For this review, take the finished solid that the model builds, in its own axes (mm). Face numbers are marked on the shaded views. A direction names the side the tool comes from. Coordinates: 2 decimals unless noted, no trailing zeros. Loops run counter-clockwise (first coordinate to the right, second up) from the corner with the lowest first, then second, coordinate; pieces in that order, holes last.
1. Take a section at A-A, the plane x = 65. Count the separate pieces of the cut face and the enclosed holes in it, then the cut area to 3 significant figures.
2. Clearance check with flat-ended pins moving along their axes: P1, Ø14.5, axis at y = 9.5, z = -78, coming from the -X side; P2, Ø1, axis at x = 55.5, y = 88, coming from the +Z side; P3, Ø4.5, axis at x = 42, y = 48, coming from the -Z side. State where each tip first meets the part, or that it passes through.
3. Take a section at B-B, the plane z = 59.5. State the section outline as (x, y) points, then the cut area to 3 significant figures.
4. Take a section at D-D, the plane z = -88. State the section outline as (x, y) points.
5. To check wall thickness, follow probe 1 along X at (y, z) = (13, 30); probe 2 along X at (y, z) = (11, -58); probe 3 along X at (y, z) = (12, -79). State the ranges of each line that lie inside material, in increasing order.
6. Machinability: for the marked faces 1, 2, 3 and 4, which of the approach directions +Z, -Z, +X, -X, +Y, -Y give a long, thin tool a straight path to every point of the face, cutting with its end or side? Answer none if there is none.
7. Take a section at C-C, the plane y = 47. State the section outline as (x, z) points, then the cut area to 3 significant figures.
8. Mouldability with a two-part tool opening along X and no side actions: class the marked faces 5, 6 and 7 as pulls with the +X half, pulls with the -X half, needs draft (parallel to the pull), parting line crosses it, or undercut.
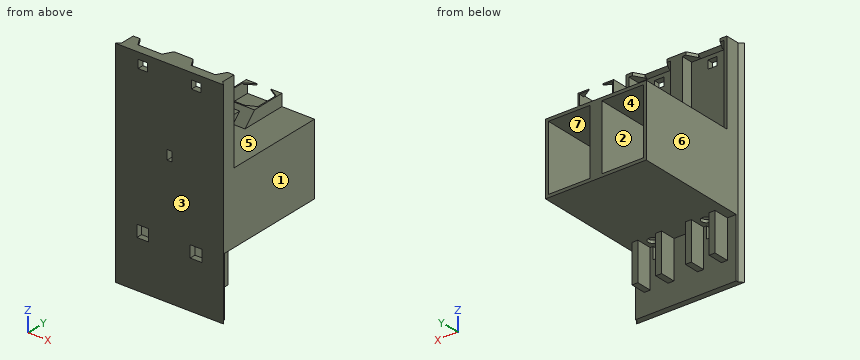
```python
from build123d import *

# Parameters (mm, degrees)
SKETCH1_W                                 = 85
SKETCH1_H                                 = 60
BOSS_EXTRUDE1_DEPTH                       = 100
CUT_EXTRUDE1_START                        = 5
SKETCH2_W                                 = 35
SKETCH2_H                                 = 55
CUT_EXTRUDE1_DEPTH                        = 95
SKETCH3_W                                 = 85
SKETCH3_H                                 = 5
BOSS_EXTRUDE2_DEPTH                       = 70
BOSS_EXTRUDE3_DEPTH                       = 10
SKETCH5_W                                 = 20
SKETCH5_H                                 = 2.5
CUT_EXTRUDE2_DEPTH                        = 7.5
SKETCH6_W                                 = 35
SKETCH6_H                                 = 12
CUT_EXTRUDE4_DEPTH                        = 57.5
CUT_EXTRUDE6_REACH                        = 186.73
SKETCH7_R                                 = 4
SKETCH9_W                                 = 85
SKETCH9_H                                 = 50
BOSS_EXTRUDE4_DEPTH                       = 5
SKETCH13_W                                = 8
SKETCH13_H                                = 7
CUT_EXTRUDE8_BUTTON_HOLES_DEPTH           = 169.374582405
BOSS_EXTRUDE5_OLED_MOUNT_DEPTH            = 10
BOSS_EXTRUDE6_OLED_MOUNT_DEPTH            = 1
BOSS_EXTRUDE7_START                       = -2.5
BOSS_EXTRUDE7_OLED_MOUNT_DEPTH            = 1
BOSS_EXTRUDE8_OLED_MOUNT_DEPTH            = 1
BOSS_EXTRUDE13_OLED_MOUNT_SUPPORT_DEPTH   = 30
CUT_EXTRUDE9_OLED_CABLE_DEPTH             = 10
CUT_EXTRUDE9_OLED_CABLE_DEPTH_BACK        = 157.553505231
SKETCH18_W                                = 4
SKETCH18_H                                = 8
BOSS_EXTRUDE12_OLED_CABLE_GUIDE_REACH     = 164.942
SKETCH20_W                                = 10
SKETCH20_H                                = 10
CUT_EXTRUDE10_SOLENOID_WIRE_HOLE_DEPTH    = 169.374582405
SKETCH21_W                                = 5
SKETCH21_H                                = 32
BOSS_EXTRUDE9_SOLENOID_SIDE_SUPPORT_DEPTH = 13
CHAMFER3_THUMB_SIZE                       = 2.5
CHAMFER5_THUMB_SIZE                       = 4.5
CHAMFER5_THUMB_SIZE2                      = 7.794228634
CHAMFER5_THUMB_PART_2_SIZE                = 4.5
CHAMFER5_THUMB_PART_2_SIZE2               = 7.794228634
CHAMFER5_THUMB_PART_3_SIZE                = 4.5
CHAMFER5_THUMB_PART_3_SIZE2               = 7.794228634
BOSS_EXTRUDE5_GUIDE_DEPTH                 = 180
SKETCH49_W                                = 10
SKETCH49_H                                = 10
BOSS_EXTRUDE14_DEPTH                      = 10
CHAMFER8_SIZE                             = 10


with BuildPart() as part:
    # Sketch1 → Boss-Extrude1 (new body)
    with BuildSketch(Plane(origin=(0, 0, 0), x_dir=(1, 0, 0), z_dir=(0, 1, 0))):
        with Locations((42.5, 30)):
            Rectangle(SKETCH1_W, SKETCH1_H)
    extrude(amount=BOSS_EXTRUDE1_DEPTH)

    # Sketch2 → Cut-Extrude1 (cut)
    with BuildSketch(Plane(origin=(0, 0, 0), x_dir=(1, 0, 0), z_dir=(0, 1, 0)).offset(CUT_EXTRUDE1_START)):
        with Locations((20, 30)):
            Rectangle(SKETCH2_W, SKETCH2_H)
        with Locations((65, 30)):
            Rectangle(SKETCH2_W, SKETCH2_H)
    extrude(amount=CUT_EXTRUDE1_DEPTH, mode=Mode.SUBTRACT)

    # Sketch3 → Boss-Extrude2 (add)
    with BuildSketch(Plane.XY):
        with Locations((42.5, 2.5)):
            Rectangle(SKETCH3_W, SKETCH3_H)
    extrude(amount=BOSS_EXTRUDE2_DEPTH)

    # Sketch4 → Boss-Extrude3 (add)
    with BuildSketch(Plane(origin=(0, 5, 0), x_dir=(1, 0, 0), z_dir=(0, 1, 0))):
        Polygon((85, 0), (82.5, 0), (82.5, -67.5), (47.5, -67.5), (47.5, 0), (37.5, 0), (37.5, -67.5), (2.5, -67.5), (2.5, 0), (0, 0), (0, -70), (85, -70), align=None)
    extrude(amount=BOSS_EXTRUDE3_DEPTH)

    # Sketch5 → Cut-Extrude2 (cut)
    with BuildSketch(Plane(origin=(0, 15, 0), x_dir=(1, 0, 0), z_dir=(0, 1, 0))):
        with Locations((20, -68.75)):
            Rectangle(SKETCH5_W, SKETCH5_H)
        with Locations((65, -68.75)):
            Rectangle(SKETCH5_W, SKETCH5_H)
    extrude(amount=-CUT_EXTRUDE2_DEPTH, mode=Mode.SUBTRACT)

    # Sketch6 → Cut-Extrude4 (cut)
    with BuildSketch(Plane.XY):
        with Locations((20, 11)):
            Rectangle(SKETCH6_W, SKETCH6_H)
        with Locations((65, 11)):
            Rectangle(SKETCH6_W, SKETCH6_H)
    extrude(amount=-CUT_EXTRUDE4_DEPTH, mode=Mode.SUBTRACT)

    # Sketch7 → Cut-Extrude6 (cut, up to next)
    with BuildSketch(Plane(origin=(0, 0, -60), x_dir=(-1, 0, 0), z_dir=(0, 0, -1)), mode=Mode.PRIVATE) as cut_extrude6_sk1:
        with Locations((-20, 11.5)):
            Circle(SKETCH7_R)
    cut_extrude6_tool1 = extrude(cut_extrude6_sk1.sketch, amount=-CUT_EXTRUDE6_REACH, mode=Mode.PRIVATE) & part.part
    # Sketch7 → Cut-Extrude6 (cut, up to next)
    with BuildSketch(Plane(origin=(0, 0, -60), x_dir=(-1, 0, 0), z_dir=(0, 0, -1)), mode=Mode.PRIVATE) as cut_extrude6_sk2:
        with Locations((-65, 11.5)):
            Circle(SKETCH7_R)
    cut_extrude6_tool2 = extrude(cut_extrude6_sk2.sketch, amount=-CUT_EXTRUDE6_REACH, mode=Mode.PRIVATE) & part.part
    add(cut_extrude6_tool1.solids().sort_by_distance((20, 11.5, -60))[0], mode=Mode.SUBTRACT)
    add(cut_extrude6_tool2.solids().sort_by_distance((65, 11.5, -60))[0], mode=Mode.SUBTRACT)

    # Sketch9 → Boss-Extrude4 (add)
    with BuildSketch(Plane(origin=(0, 0, 0), x_dir=(1, 0, 0), z_dir=(0, 1, 0))):
        with Locations((42.5, 85)):
            Rectangle(SKETCH9_W, SKETCH9_H)
    extrude(amount=BOSS_EXTRUDE4_DEPTH)

    # Sketch13 → Cut-Extrude8 (Button Holes) (cut, through all)
    with BuildSketch(Plane(origin=(0, 5, 0), x_dir=(1, 0, 0), z_dir=(0, 1, 0))):
        with Locations((20, -61)):
            Rectangle(SKETCH13_W, SKETCH13_H)
        with Locations((65, -61)):
            Rectangle(SKETCH13_W, SKETCH13_H)
    extrude(amount=-CUT_EXTRUDE8_BUTTON_HOLES_DEPTH, mode=Mode.SUBTRACT)

    # Sketch14 → Boss-Extrude5 (OLED Mount) (add)
    with BuildSketch(Plane.XY):
        Polygon((27.5, 100), (28.5, 100), (28.5, 72), (56.5, 72), (56.5, 100), (57.5, 100), (57.5, 71), (52.172712592, 71), (32.827287408, 71), (27.5, 71), align=None)
    extrude(amount=BOSS_EXTRUDE5_OLED_MOUNT_DEPTH)

    # Sketch15 → Boss-Extrude6 (OLED Mount) (add)
    with BuildSketch(Plane.XY.offset(10)):
        Polygon((28.5, 72), (36.5, 72), (28.5, 76), align=None)
        Polygon((56.5, 76), (56.5, 72), (48.5, 72), align=None)
    extrude(amount=-BOSS_EXTRUDE6_OLED_MOUNT_DEPTH)

    # Sketch15<2> → Boss-Extrude7 (OLED Mount) (add)
    with BuildSketch(Plane.XY.offset(10).offset(BOSS_EXTRUDE7_START)):
        Polygon((28.5, 72), (36.5, 72), (28.5, 76), align=None)
        Polygon((56.5, 76), (56.5, 72), (48.5, 72), align=None)
    extrude(amount=-BOSS_EXTRUDE7_OLED_MOUNT_DEPTH)

    # Sketch17 → Boss-Extrude8 (OLED Mount) (add)
    with BuildSketch(Plane.XY.offset(10)):
        Polygon((56.5, 95), (56.5, 100), (48.5, 100), align=None)
        Polygon((28.5, 100), (36.5, 100), (28.5, 95), align=None)
    extrude(amount=-BOSS_EXTRUDE8_OLED_MOUNT_DEPTH)

    # Sketch32 → Boss-Extrude13 OLED Mount Support) (add)
    with BuildSketch(Plane.ZY.offset(-27.5)):
        Polygon((0, 71), (10, 71), (0, 61), align=None)
    extrude(amount=-BOSS_EXTRUDE13_OLED_MOUNT_SUPPORT_DEPTH)

    # Sketch18 → Cut-Extrude9 (OLED Cable) (cut, two sides: drawn at the far end of the back side and taken through both)
    with BuildSketch(Plane(origin=(0, 72, 0), x_dir=(1, 0, 0), z_dir=(0, 1, 0)).offset(-CUT_EXTRUDE9_OLED_CABLE_DEPTH_BACK)):
        with Locations((42.5, -1)):
            Rectangle(SKETCH18_W, SKETCH18_H)
    extrude(amount=CUT_EXTRUDE9_OLED_CABLE_DEPTH + CUT_EXTRUDE9_OLED_CABLE_DEPTH_BACK, mode=Mode.SUBTRACT)

    # Boss-Extrude12 (OLED Cable Guide): up to this plane
    boss_extrude12_oled_cable_guide_end = Plane(origin=(57.5, 71, 10), z_dir=(0, -0.7071067811865475, 0.7071067811865476))
    # Sketch31 → Boss-Extrude12 (OLED Cable Guide) (add, up to the surface)
    with BuildSketch(Plane(origin=(0, 15, 0), x_dir=(1, 0, 0), z_dir=(0, 1, 0)), mode=Mode.PRIVATE) as boss_extrude12_oled_cable_guide_sk1:
        Polygon((37.5, 0), (40.5, 0), (40.5, -5), (44.5, -5), (44.5, 0), (47.5, 0), (47.5, -7), (37.5, -7), align=None)
    boss_extrude12_oled_cable_guide_tool1 = split(extrude(boss_extrude12_oled_cable_guide_sk1.sketch, amount=BOSS_EXTRUDE12_OLED_CABLE_GUIDE_REACH, mode=Mode.PRIVATE), bisect_by=boss_extrude12_oled_cable_guide_end, keep=Keep.BOTH, mode=Mode.PRIVATE)
    add(boss_extrude12_oled_cable_guide_tool1.solids().sort_by_distance((39, 15, 0.122066))[0])

    # Sketch20 → Cut-Extrude10 (Solenoid Wire Hole) (cut, through all)
    with BuildSketch(Plane(origin=(0, 5, 0), x_dir=(1, 0, 0), z_dir=(0, 1, 0))):
        with Locations((65, 65)):
            Rectangle(SKETCH20_W, SKETCH20_H)
        with Locations((20, 65)):
            Rectangle(SKETCH20_W, SKETCH20_H)
    extrude(amount=-CUT_EXTRUDE10_SOLENOID_WIRE_HOLE_DEPTH, mode=Mode.SUBTRACT)

    # Sketch21 → Boss-Extrude9 (Solenoid Side Support) (add)
    with BuildSketch(Plane(origin=(0, 5, 0), x_dir=(1, 0, 0), z_dir=(0, 1, 0))):
        with Locations((75, 76)):
            Rectangle(SKETCH21_W, SKETCH21_H)
        with Locations((55, 76)):
            Rectangle(SKETCH21_W, SKETCH21_H)
        with Locations((30, 76)):
            Rectangle(SKETCH21_W, SKETCH21_H)
        with Locations((10, 76)):
            Rectangle(SKETCH21_W, SKETCH21_H)
    extrude(amount=BOSS_EXTRUDE9_SOLENOID_SIDE_SUPPORT_DEPTH)

    # Chamfer3 (Thumb)
    chamfer3_thumb_edges = [part.edges().sort_by_distance(p)[0] for p in [
        (20, 7.5, 67.5),
        (65, 7.5, 67.5),
    ]]
    chamfer(chamfer3_thumb_edges, length=CHAMFER3_THUMB_SIZE - 0.0001)  # a hair under: the kernel refuses the full size

    # Chamfer5 (Thumb)
    chamfer5_thumb_edges = [part.edges().sort_by_distance(p)[0] for p in [
        (75, 15, 68.75),
    ]]
    chamfer5_thumb_side = [part.faces().sort_by_distance(p)[0] for p in [
        (83.266129032, 15, 38.266129032),
    ]]
    chamfer(chamfer5_thumb_edges, length=CHAMFER5_THUMB_SIZE, length2=CHAMFER5_THUMB_SIZE2, reference=chamfer5_thumb_side[0])

    # Chamfer5 (Thumb) part 2
    chamfer5_thumb_part_2_edges = [part.edges().sort_by_distance(p)[0] for p in [
        (55, 15, 68.75),
        (30, 15, 68.75),
    ]]
    chamfer5_thumb_part_2_side = [part.faces().sort_by_distance(p)[0] for p in [
        (42.5, 15, 40.199438202),
    ]]
    chamfer(chamfer5_thumb_part_2_edges, length=CHAMFER5_THUMB_PART_2_SIZE, length2=CHAMFER5_THUMB_PART_2_SIZE2, reference=chamfer5_thumb_part_2_side[0])

    # Chamfer5 (Thumb) part 3
    chamfer5_thumb_part_3_edges = [part.edges().sort_by_distance(p)[0] for p in [
        (10, 15, 68.75),
    ]]
    chamfer5_thumb_part_3_side = [part.faces().sort_by_distance(p)[0] for p in [
        (1.733870968, 15, 38.266129032),
    ]]
    chamfer(chamfer5_thumb_part_3_edges, length=CHAMFER5_THUMB_PART_3_SIZE, length2=CHAMFER5_THUMB_PART_3_SIZE2, reference=chamfer5_thumb_part_3_side[0])

    # Sketch37 → Boss-Extrude5 (Guide) (add, through all)
    with BuildSketch(Plane.XY.offset(70)):
        Polygon((85, 0), (88, 0), (85, 3), align=None)
        Polygon((0, 0), (-3, 0), (0, 3), align=None)
    extrude(amount=-BOSS_EXTRUDE5_GUIDE_DEPTH)

    # Sketch49 → Boss-Extrude14 (add)
    with BuildSketch(Plane(origin=(0, 15, 0), x_dir=(1, 0, 0), z_dir=(0, 1, 0))):
        with Locations((42.5, -12)):
            Rectangle(SKETCH49_W, SKETCH49_H)
    extrude(amount=BOSS_EXTRUDE14_DEPTH)

    # Chamfer8
    chamfer8_edges = [part.edges().sort_by_distance(p)[0] for p in [
        (42.5, 25, 17),
    ]]
    chamfer(chamfer8_edges, length=CHAMFER8_SIZE - 0.0001)  # a hair under: the kernel refuses the full size


solid = part.part
```
Results list:
1. separate pieces: 5
1. enclosed holes: 0
1. area: 1,240 mm2
2. P1: stops at x = -0.75
2. P2: stops at z = 0
2. P3: stops at z = -60
3. outline: (-3, 0) - (16, 0) - (16, 5) - (2.5, 5) - (2.5, 15) - (0, 15) - (0, 3) - close; (24, 0) - (61, 0) - (61, 5) - (47.5, 5) - (47.5, 15) - (37.5, 15) - (37.5, 5) - (24, 5) - close; (69, 0) - (88, 0) - (85, 3) - (85, 15) - (82.5, 15) - (82.5, 5) - (69, 5) - close
3. area: 504 mm2
4. outline: (-3, 0) - (88, 0) - (85, 3) - (85, 5) - (77.5, 5) - (77.5, 18) - (72.5, 18) - (72.5, 5) - (57.5, 5) - (57.5, 18) - (52.5, 18) - (52.5, 5) - (32.5, 5) - (32.5, 18) - (27.5, 18) - (27.5, 5) - (12.5, 5) - (12.5, 18) - (7.5, 18) - (7.5, 5) - (0, 5) - (0, 3) - close
5. probe 1: x = 0 to 2.5, 37.5 to 47.5, 82.5 to 85
5. probe 2: x = 0 to 16.03, 23.97 to 61.03, 68.97 to 85
5. probe 3: x = 7.5 to 12.5, 27.5 to 32.5, 52.5 to 57.5, 72.5 to 77.5
6. face 1: +Z, -Z, +X, +Y
6. face 2: none
6. face 3: +Z, -Z, +X, -X, -Y
6. face 4: +Y
7. outline: (0, -60) - (85, -60) - (85, 0) - (47.5, 0) - (47.5, 7) - (37.5, 7) - (37.5, 0) - (0, 0) - close; hole (2.5, -57.5) - (37.5, -57.5) - (37.5, -2.5) - (2.5, -2.5) - close; hole (40.5, -3) - (44.5, -3) - (44.5, 5) - (40.5, 5) - close; hole (47.5, -57.5) - (82.5, -57.5) - (82.5, -2.5) - (47.5, -2.5) - close
7. area: 1,290 mm2
8. face 5: needs draft
8. face 6: pulls with the -X half
8. face 7: undercut
